Design review of the part shown in the three views and the two pictorial views. Dimensions are in mm from the part's minimum x, y and z. Coordinates: 2 decimals unless noted, no trailing zeros. Loops run counter-clockwise (first coordinate to the right, second up) from the corner with the lowest first, then second, coordinate; pieces in that order, holes last.
Q1. Add section C-C on z = 67.5. Give the boundary of the cut face in (x, y), and give its area (3 significant figures).
Q2. Add section A-A on y = 1.75. Give the number of separate pieces and of enclosed holes in the cut face, and give its area (3 significant figures).
Q3. For P1, Ø3, axis at x = 2, y = 3, coming from the +Z side; P2, Ø1, axis at y = 5.5, z = 36, coming from the -X side; P3, Ø1.9, axis at x = 238.5, y = 3, coming from the +Z side; P4, Ø2.5, axis at x = 238.125, z = 25.4, coming from the +Y side, all flat-tipped, find the tip position at first contact; note any pin that passes through.
Q4. Add section B-B on z = 17.5. Give the boundary of the cut face in (x, y).
Q5. Wall thickness on probe 1 along X at (y, z) = (5, 25); probe 2 along X at (y, z) = (3.25, 68); probe 3 along X at (y, z) = (6, 55.5): over which ranges is each line inside the solid? List them lowest first.
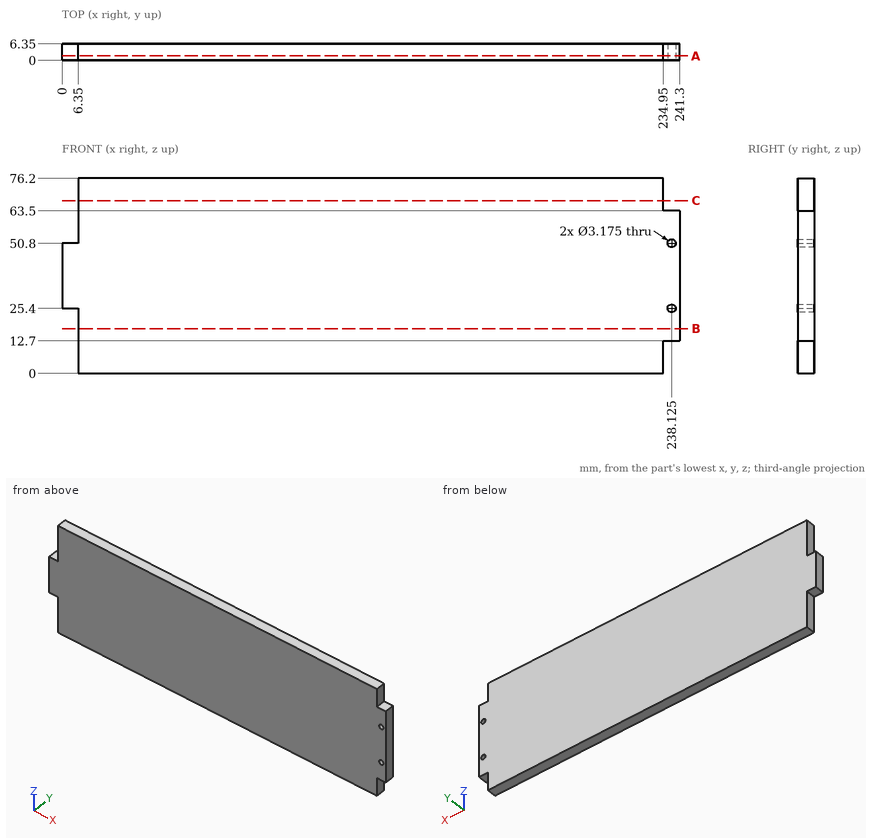
Entries:
1. outline: (6.35, 0) - (234.95, 0) - (234.95, 6.35) - (6.35, 6.35) - close
1. area: 1,450 mm2
2. separate pieces: 1
2. enclosed holes: 2
2. area: 17,900 mm2
3. P1: stops at z = 50.8
3. P2: stops at x = 0
3. P3: stops at z = 63.5
3. P4: passes through
4. outline: (6.35, 0) - (241.3, 0) - (241.3, 6.35) - (6.35, 6.35) - close
5. probe 1: x = 6.35 to 236.59, 239.66 to 241.3
5. probe 2: x = 6.35 to 234.95
5. probe 3: x = 6.35 to 241.3
